Read the model definition and answer for the solid it produces. Units are mm, in the model's axes. Face numbers are marked on the shaded views. A direction names the side the tool comes from. Coordinates: 2 decimals unless noted, no trailing zeros. Write each loop counter-clockwise with the first axis right and the second up, starting at its lowest first coordinate (ties: lowest second). Pieces come first, ordered by that corner, then holes.
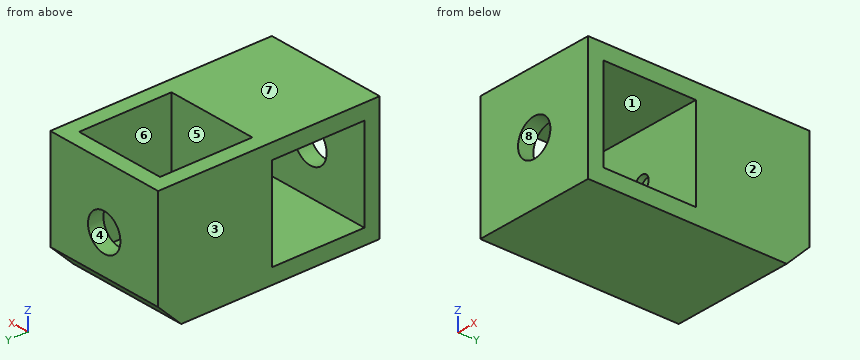
from build123d import *

# Parameters (mm, degrees)
SKETCH2_W               = 40
SKETCH2_H               = 72
BOSS_EXTRUDE1_DEPTH     = 20
SKETCH3_W               = 30
SKETCH3_H               = 30
CUT_EXTRUDE1_DEPTH      = 35
CUT_EXTRUDE2_DEPTH      = 46.782092569
CUT_EXTRUDE2_DEPTH_BACK = 46.782092569
SKETCH4_W               = 30
SKETCH4_H               = 30
CHAMFER1_SIZE           = 7.5
CUT_EXTRUDE3_DEPTH      = 46.782092569
CUT_EXTRUDE3_DEPTH_BACK = 46.782092569
SKETCH5_R               = 6
SKETCH6_R               = 6
SKETCH6_R_2             = 2.5
BOSS_EXTRUDE2_DEPTH     = 1


with BuildPart() as part:
    # Sketch2 → Boss-Extrude1 (new, symmetric)
    with BuildSketch(Plane.XY):
        Rectangle(SKETCH2_W, SKETCH2_H)
    extrude(amount=BOSS_EXTRUDE1_DEPTH, both=True)

    # Sketch3 → Cut-Extrude1 (cut)
    with BuildSketch(Plane.XY.offset(20)):
        with Locations((0, 16)):
            Rectangle(SKETCH3_W, SKETCH3_H)
    extrude(amount=-CUT_EXTRUDE1_DEPTH, mode=Mode.SUBTRACT)

    # Sketch4 → Cut-Extrude2 (cut, two sides: drawn at the far end of the back side and taken through both)
    with BuildSketch(Plane(origin=(0, 0, 0), x_dir=(0, 0, -1), z_dir=(1, 0, 0)).offset(-CUT_EXTRUDE2_DEPTH_BACK)):
        with Locations((0, -16)):
            Rectangle(SKETCH4_W, SKETCH4_H)
    extrude(amount=CUT_EXTRUDE2_DEPTH + CUT_EXTRUDE2_DEPTH_BACK, mode=Mode.SUBTRACT)

    # Chamfer1
    chamfer1_edges = [part.edges().sort_by_distance(p)[0] for p in [
        (0, 36, -20),
    ]]
    chamfer(chamfer1_edges, length=CHAMFER1_SIZE)

    # Sketch5 → Cut-Extrude3 (cut, two sides: drawn at the far end of the back side and taken through both)
    with BuildSketch(Plane(origin=(0, 0, 0), x_dir=(1, 0, 0), z_dir=(0, 1, 0)).offset(-CUT_EXTRUDE3_DEPTH_BACK)):
        with Locations(Location((0, 0, 0), (0, 0, 270))):
            Circle(SKETCH5_R)
    extrude(amount=CUT_EXTRUDE3_DEPTH + CUT_EXTRUDE3_DEPTH_BACK, mode=Mode.SUBTRACT)

    # Sketch6 → Boss-Extrude2 (add, symmetric)
    with BuildSketch(Plane(origin=(0, 0, 0), x_dir=(1, 0, 0), z_dir=(0, 1, 0))):
        with Locations(Location((0, 0, 0), (0, 0, 270))):
            Circle(SKETCH6_R)
        with Locations(Location((0, 0, 0), (0, 0, 270))):
            Circle(SKETCH6_R_2, mode=Mode.SUBTRACT)
    extrude(amount=BOSS_EXTRUDE2_DEPTH, both=True)


solid = part.part
Item 1: The part is cut by section C-C (y = -7). Give the vertices of the cut face in (x, z).
Item 2: The part is cut by section D-D (x = -16.5). Give the vertices of the cut face in (y, z).
Item 3: For the marked faces 1, 2, 3, 4 and 5, determine the directions among +Z, -Z, +X, -X, +Y, -Y from which every point of the face is accessible in a straight line to the end or side of a thin tool.
Item 4: Determine the mould class of the marked faces 6, 7 and 8 for opening direction Z: +Z half, -Z half, draft (parallel to the pull), parting line (faces both ways), or undercut.
Item 5: Given pin 1 (19 mm diameter, centred on x = 0, z = 0, fed in from -Y); pin 2 (15 mm diameter, centred on x = -1, y = 21.5, fed in from +Z); pin 3 (3 mm diameter, centred on x = 0, z = 0, fed in from -Y), each flat-ended and moving along its own axis, determine where each tip first touches the part or whether it passes through.
Item 6: Find the intervals of material crossed by probe 1 along Y at (x, z) = (1, 11.5); probe 2 along Z at (x, y) = (-16.5, -26); probe 3 along Y at (x, z) = (12, 16), in increasing order.
Item 7: The part is cut by section A-A (z = -10). Give the vertices of the cut face in (x, y).
Item 8: The part is cut by section B-B (z = 0). Give the vertices of the cut face in (x, y).
Answer:
1. outline: (-20, -20) - (20, -20) - (20, -15) - (-20, -15) - close; (-20, 15) - (20, 15) - (20, 20) - (-20, 20) - close
2. outline: (-36, -20) - (28.5, -20) - (36, -12.5) - (36, 20) - (-36, 20) - close; hole (-31, -15) - (-1, -15) - (-1, 15) - (-31, 15) - close
3. face 1: +X, -X
3. face 2: +Z, -Z, +X, +Y, -Y
3. face 3: +Z, -Z, -X, +Y, -Y
3. face 4: +Y
3. face 5: +Z
4. face 6: draft
4. face 7: +Z half
4. face 8: undercut
5. pin 1: stops at y = -36
5. pin 2: stops at z = -15
5. pin 3: passes through
6. probe 1: y = -36 to -31, -1 to 1, 31 to 36
6. probe 2: z = -20 to -15, 15 to 20
6. probe 3: y = -36 to 1, 31 to 36
7. outline: (-20, -36) - (20, -36) - (20, -31) - (-20, -31) - close; (-20, -1) - (20, -1) - (20, 36) - (-20, 36) - close; hole (-15, 1) - (15, 1) - (15, 31) - (-15, 31) - close
8. outline: (-20, -36) - (-6, -36) - (-6, -31) - (-20, -31) - close; (-20, -1) - (-2.5, -1) - (-2.5, 1) - (-15, 1) - (-15, 31) - (-6, 31) - (-6, 36) - (-20, 36) - close; (2.5, -1) - (20, -1) - (20, 36) - (6, 36) - (6, 31) - (15, 31) - (15, 1) - (2.5, 1) - close; (6, -36) - (20, -36) - (20, -31) - (6, -31) - close
